Study the drawing (mm; zero at the part's minimum x, y, z) and answer. Coordinates: 2 decimals unless noted, no trailing zeros. Loops run counter-clockwise (first coordinate to the right, second up) from the corner with the lowest first, then second, coordinate; pieces in that order, holes last. Notation, with made-up numbers: (72.5, 52.5) -> (109.5, 52.5) arc R19 cw to (109.5, 83.5) -> close; hole circle Ø9 at (-18, 49.5). An arc over 180 degrees is marked (long way). One line per question, with ' | ' between items.
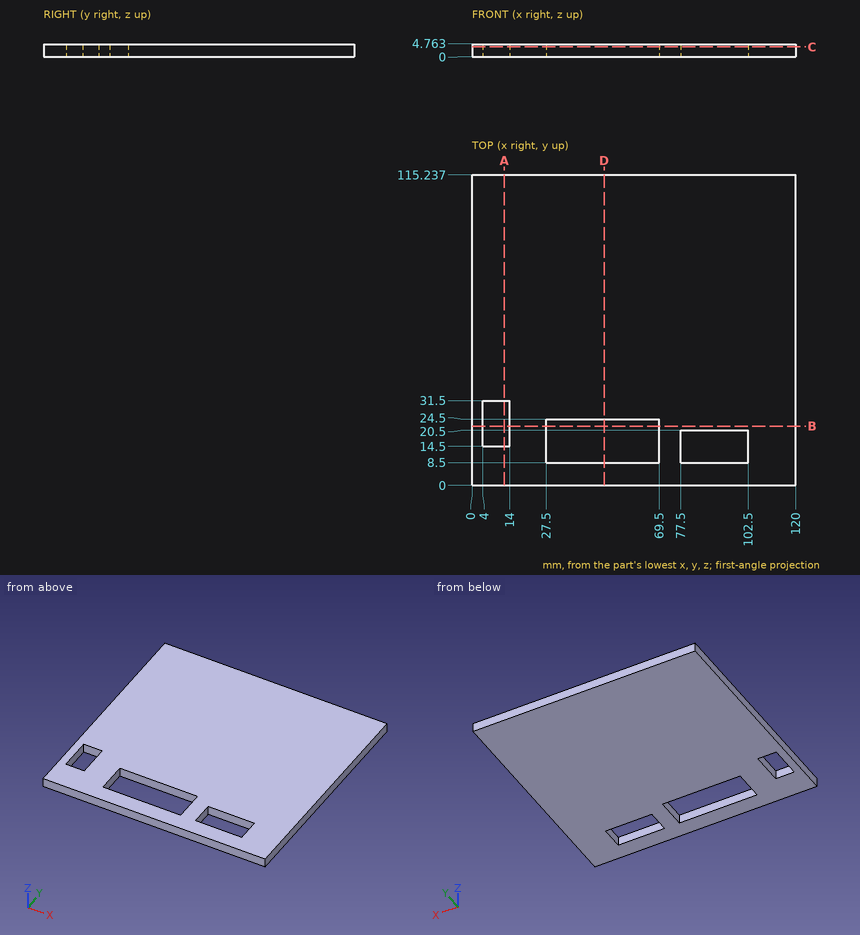
1) Find the intervals of material crossed by line 1 along Y through (x, z) = (37, 1.4); line 2 along Y through (x, z) = (87, 2.6); line 3 along X through (y, z) = (24, 0.95), in increasing order.
Check values:
line 1: y = 0 to 8.5, 24.5 to 115.24 | line 2: y = 0 to 8.5, 20.5 to 115.24 | line 3: x = 0 to 4, 14 to 27.5, 69.5 to 120
2) Find section D-D (x = 49). Write down the section's boundary in (y, z).
Check values:
outline: (0, 0) -> (8.5, 0) -> (8.5, 4.76) -> (0, 4.76) -> close; (24.5, 0) -> (115.24, 0) -> (115.24, 4.76) -> (24.5, 4.76) -> close
3) Find section A-A (x = 12). Write down the section's boundary in (y, z).
Check values:
outline: (0, 0) -> (14.5, 0) -> (14.5, 4.76) -> (0, 4.76) -> close; (31.5, 0) -> (115.24, 0) -> (115.24, 4.76) -> (31.5, 4.76) -> close
4) Find section B-B (y = 22). Write down the section's boundary in (x, z).
Check values:
outline: (0, 0) -> (4, 0) -> (4, 4.76) -> (0, 4.76) -> close; (14, 0) -> (27.5, 0) -> (27.5, 4.76) -> (14, 4.76) -> close; (69.5, 0) -> (120, 0) -> (120, 4.76) -> (69.5, 4.76) -> close
5) Find section C-C (z = 3.7). Write down the section's boundary in (x, y), plus the area to 3 significant figures.
Check values:
outline: (0, 0) -> (120, 0) -> (120, 115.24) -> (0, 115.24) -> close; hole (4, 14.5) -> (14, 14.5) -> (14, 31.5) -> (4, 31.5) -> close; hole (27.5, 8.5) -> (69.5, 8.5) -> (69.5, 24.5) -> (27.5, 24.5) -> close; hole (77.5, 8.5) -> (102.5, 8.5) -> (102.5, 20.5) -> (77.5, 20.5) -> close | area: 12,700 mm^2
